The listing builds one solid part. Answer for the finished solid, in the listing's coordinates (mm). Coordinates: 2 decimals unless noted, no trailing zeros. Order: outer loops, then holes, each group sorted by start corner. A loop starts at its lowest first (then second) coordinate and runs counter-clockwise, first axis right, second up. Notation, with made-up numbers: (84.25, 25) -> (108.25, 25) arc R21 ccw to (108.25, 37) -> close; hole circle Ø9 at (-36.5, -8.5). An arc over 180 degrees is marked (long way). Answer in a Markdown table with one row per item. Add a question column.
```python
from build123d import *

# Parameters (mm, degrees)
SKETCH1_W                    = 270
SKETCH1_H                    = 1965
MAIN_PLATE_EXTRUDE_DEPTH     = 5
MOTOR_MOUNT_CUT_DEPTH        = 992.7440446
MOTOR_MOUNT_CUT_DEPTH_BACK   = 992.7440446
SKETCH2_W                    = 221
SKETCH2_H                    = 5
OUTPUT_SHAFT_SLOT_DEPTH      = 992.7440446
OUTPUT_SHAFT_SLOT_DEPTH_BACK = 992.7440446


with BuildPart() as part:
    # Sketch1 → Main plate extrude (new body)
    with BuildSketch(Plane.XY):
        Rectangle(SKETCH1_W, SKETCH1_H)
    extrude(amount=MAIN_PLATE_EXTRUDE_DEPTH)

    # Sketch2 → Motor mount cut (cut, two sides: drawn at the far end of the back side and taken through both)
    with BuildSketch(Plane.XY.offset(5).offset(-MOTOR_MOUNT_CUT_DEPTH_BACK)):
        with Locations((-2.5, -980)):
            Rectangle(SKETCH2_W, SKETCH2_H)
    extrude(amount=MOTOR_MOUNT_CUT_DEPTH + MOTOR_MOUNT_CUT_DEPTH_BACK, mode=Mode.SUBTRACT)

    # Sketch3 → Output shaft slot (cut, two sides: drawn at the far end of the back side and taken through both)
    with BuildSketch(Plane.XY.offset(5).offset(-OUTPUT_SHAFT_SLOT_DEPTH_BACK)):
        with BuildLine():
            Line((-85, 750), (-85, -750))
            ThreePointArc((-85, -750), (-95, -760), (-105, -750))
            Line((-105, -750), (-105, 750))
            ThreePointArc((-105, 750), (-95, 760), (-85, 750))
        make_face()
    extrude(amount=OUTPUT_SHAFT_SLOT_DEPTH + OUTPUT_SHAFT_SLOT_DEPTH_BACK, mode=Mode.SUBTRACT)


solid = part.part
```
Q1. Straight lines are drawn through the part: line 1 (X direction, y = 210, z = 3.7); line 2 (Y direction, x = 28, z = 0.7); line 3 (Y direction, x = -102.5, z = 1.35). For each, find the intervals that lie inside material, in ascending order.
Q2. A cutting plane is placed at A-A (z = 4.15). Determine the outline of the cut face in (x, y).
Q3. A cutting plane is placed at B-B (y = -195.5). Determine the outline of the cut face in (x, z).
Returned:
| question | item | result |
|---|---|---|
| 1 | line 1 | x = -135 to -105, -85 to 135 |
| 1 | line 2 | y = -977.5 to 982.5 |
| 1 | line 3 | y = -977.5 to -756.61, 756.61 to 982.5 |
| 2 | outline | (-135, -982.5) -> (-113, -982.5) -> (-113, -977.5) -> (108, -977.5) -> (108, -982.5) -> (135, -982.5) -> (135, 982.5) -> (-135, 982.5) -> close; hole (-105, -750) arc R10 ccw to (-85, -750) -> (-85, 750) arc R10 ccw to (-105, 750) -> close |
| 3 | outline | (-135, 0) -> (-105, 0) -> (-105, 5) -> (-135, 5) -> close; (-85, 0) -> (135, 0) -> (135, 5) -> (-85, 5) -> close |
